Could you check a few things on this model? Use its own coordinates, in mm. A direction names the side the tool comes from. Coordinates: 2 decimals unless noted, no trailing zeros. Loops run counter-clockwise (first coordinate to the right, second up) from the corner with the lowest first, then second, coordinate; pieces in that order, holes last. Notation, with made-up numbers: (-23, 2.25) -> (7, 2.25) arc R19 ccw to (7, 7.25) -> close; hole circle Ø8 at (9, 66.25). An arc over 180 degrees is marked (long way). One line per question, with ' | ' between items.
from build123d import *

# Parameters (mm, degrees)
EXTRU_MINCE1_DEPTH      = 118
ESQUISSE2_R             = 2.5
ENL_V_MAT_EXTRU_1_DEPTH = 4
ESQUISSE3_R             = 1.5
ENL_V_MAT_EXTRU_2_DEPTH = 4
CHANFREIN1_SIZE         = 25


with BuildPart() as part:
    # Esquisse1 → Extru.-Mince1 (new body)
    with BuildSketch(Plane.XY):
        Polygon((0, 15.5), (0, 0), (27.5, 0), (27.5, 1.5), (1.5, 1.5), (1.5, 15.5), align=None)
    extrude(amount=EXTRU_MINCE1_DEPTH)

    # Esquisse2 → Enlèv. mat.-Extru.1 (cut)
    with BuildSketch(Plane.ZY):
        with Locations(Location((9, 9, 0), (0, 0, 270))):
            Circle(ESQUISSE2_R)
        with Locations(Location((109, 9, 0), (0, 0, 90))):
            Circle(ESQUISSE2_R)
    extrude(amount=-ENL_V_MAT_EXTRU_1_DEPTH, mode=Mode.SUBTRACT)

    # Esquisse3 → Enlèv. mat.-Extru.2 (cut)
    with BuildSketch(Plane.XZ):
        with Locations(Location((15.771636742, 30.664864187, 0), (0, 0, 270))):
            Circle(ESQUISSE3_R)
        with Locations(Location((15.771636742, 87.335135813, 0), (0, 0, 90))):
            Circle(ESQUISSE3_R)
    extrude(amount=-ENL_V_MAT_EXTRU_2_DEPTH, mode=Mode.SUBTRACT)

    # Chanfrein1
    chanfrein1_edges = [part.edges().sort_by_distance(p)[0] for p in [
        (27.5, 0.75, 0),
        (27.5, 0.75, 118),
    ]]
    chamfer(chanfrein1_edges, length=CHANFREIN1_SIZE)


solid = part.part
1) If we section it at A-A on y = 9: Please give me the cut outline in (x, z), and give its area (3 significant figures).
Data:
outline: (0, 0) -> (1.5, 0) -> (1.5, 6.5) -> (0, 6.5) -> close; (0, 11.5) -> (1.5, 11.5) -> (1.5, 106.5) -> (0, 106.5) -> close; (0, 111.5) -> (1.5, 111.5) -> (1.5, 118) -> (0, 118) -> close | area: 162 mm²
2) On a 3-axis mill with a long thin cutter (end or side, diameter ignored), from which of +Z, -Z, +X, -X, +Y, -Y can I reach the whole of each face in a straight line? I mean faces 4 (the face through (15, 1.5, 58)), 5 (the face through (1, 8, 118)). Say none if no direction works.
Data:
face 4: +Z, -Z, +X, +Y | face 5: +Z, +X, -X, +Y, -Y
3) I'm going to push flat-ended pins straight in: pin 1 Ø3 at (x, z) = (15.5, 17) entering from +Y; pin 2 Ø4 at (y, z) = (9, 109) entering from -X; pin 3 Ø8 at (y, z) = (7, 78) entering from +X; pin 4 Ø8 at (x, y) = (13, 2) entering from -Z. Where does each tip first touch, or does it pass through?
Data:
pin 1: y = 1.5 | pin 2: through | pin 3: x = 1.5 | pin 4: z = 6.53
4) If we section it at C-C on x = 22: Please give me the cut outline in (y, z).
Data:
outline: (0, 19.5) -> (1.5, 19.5) -> (1.5, 98.5) -> (0, 98.5) -> close
5) If we section it at B-B on z = 9: Please give me the cut outline in (x, y).
Data:
outline: (0, 0) -> (11.5, 0) -> (11.5, 1.5) -> (1.5, 1.5) -> (1.5, 6.5) -> (0, 6.5) -> close; (0, 11.5) -> (1.5, 11.5) -> (1.5, 15.5) -> (0, 15.5) -> close
6) We'd pull the mould along Y, two halves only. Please class faces 1 (the face through (0.74, 9.54, 6.56)), 2 (the face through (14, 0, 58)), 3 (the face through (15.2, 0.7, 12.7)): pulls with the +Y half, pulls with the -Y half, needs draft (parallel to the pull), parting line crosses it, or undercut.
Data:
face 1: undercut | face 2: pulls with the -Y half | face 3: needs draft
7) If we section it at D-D on z = 42: Please give me the cut outline in (x, y).
Data:
outline: (0, 0) -> (27.5, 0) -> (27.5, 1.5) -> (1.5, 1.5) -> (1.5, 15.5) -> (0, 15.5) -> close
8) I need wall thicknesses on line 1 along Z through (x, y) = (1.1, 9); line 2 along X through (y, z) = (6.25, 97). Which ranges of each line are inside material? Lowest first, please. Write a range as from..to.
Data:
line 1: 0..6.5, 11.5..106.5, 111.5..118 | line 2: 0..1.5
